Autodesk Inventor part; units mm, degrees
ref_plane "Work Plane1" through (23, 0, 25.5) normal (1, 0, 0) x (0, 0, -1)
ref_plane "YZ Plane" through (0, 0, 0) normal (1, 0, 0) x (0, 1, 0)
ref_plane "XZ Plane" through (0, 0, 0) normal (0, 1, 0) x (-1, 0, 0)
sketch "Sketch1" plane through (0, 0, 0) normal (0, 1, 0) x (-1, 0, 0)
  line L0 (23, 25.5) -> (-23, 25.5)
  line L1 (-23, 25.5) -> (-23, -25.5)
  line L2 (-23, -25.5) -> (23, -25.5)
  line L3 (23, -25.5) -> (23, 25.5)
  point P0 (0, 0)
  point P1 (-23, 0)
  point P2 (23, 0)
  point P3 (0, 25.5)
  point P4 (0, -25.5)
  dimension "d0" = 46
  dimension "d1" = 51
extrude "Extrusion1" add sketch "Sketch1" along normal blind 3
sketch "Sketch2" plane through (0, 3, 0) normal (0, 1, 0) x (1, 0, 0)
  line L0 (-23, -25.5) -> (23, -25.5)
  line L1 (23, 25.5) -> (-23, 25.5)
  line L2 (-23, 25.5) -> (-23, -25.5)
  line L3 (23, -25.5) -> (23, 25.5)
  point P0 (0, 0)
  point P1 (-15, -17.5)
  point P2 (-15, 17.5)
  point P3 (15, -17.5)
  point P4 (15, 17.5)
  dimension "d4" = 8
  dimension "d5" = 8
  dimension "d6" = 8
  dimension "d7" = 8
  dimension "d8" = 8
  dimension "d9" = 8
  dimension "d10" = 8
  dimension "d11" = 8
hole "Hole1" at (-15, 3, 17.5) at (-15, 3, -17.5) at (15, 3, 17.5) at (15, 3, -17.5) direction (0, -1, 0) diameter 2 end through all
ref_plane "Work Plane1" through (23, 0, 25.5) normal (1, 0, 0) x (0, 0, -1)
sketch "Sketch3" plane through (23, 0, 25.5) normal (1, 0, 0) x (0, 0, -1)
  line L0 (25.5, 0) -> (25.5, 200)
  line L1 (60.5, 78.2142) -> (-9.5, 78.2142)
  line L2 (51, 3) -> (0, 3)
  line L3 (0, 3) -> (51, 3)
  line L4 (60.5, 78.2142) -> (60.5, 38.2142)
  line L5 (-9.5, 78.2142) -> (-9.5, 38.2142)
  line L6 (-9.5, 38.2142) -> (0, 3)
  line L7 (60.5, 38.2142) -> (51, 3)
  point P0 (25.5, 78.2142)
  point P1 (25.5, 3)
  point P2 (25.5, 3)
  dimension "d19" = 200
  dimension "d20" = 70
  dimension "d23" = 40
  dimension "d24" = 40
extrude "Extrusion3" add sketch "Sketch3" against normal blind 3
sketch "Sketch4" plane through (20, 0, 25.5) normal (-1, 0, 0) x (0, 0, 1)
  line L0 (-51, 3) -> (0, 3)
  line L1 (-60.5, 78.2142) -> (-60.5, 38.2142)
  line L2 (-51, 3) -> (-60.5, 38.2142)
  line L3 (9.5, 78.2142) -> (-60.5, 78.2142)
  line L4 (-60.5, 38.2142) -> (-60.5, 78.2142)
  line L5 (9.5, 38.2142) -> (9.5, 78.2142)
  line L6 (-60.5, 78.2142) -> (9.5, 78.2142)
  line L7 (0, 3) -> (9.5, 38.2142)
  line L8 (9.5, 78.2142) -> (9.5, 38.2142)
  line L9 (9.5, 38.2142) -> (0, 3)
  line L10 (-47.8927, 3) -> (-57.5, 38.6118)
  line L11 (-57.5, 38.6118) -> (-57.5, 75.2142)
  line L12 (-57.5, 75.2142) -> (6.5, 75.2142)
  line L13 (6.5, 75.2142) -> (6.5, 38.6118)
  line L14 (6.5, 38.6118) -> (-3.1073, 3)
  point P0 (-25.5, 0)
  dimension "d27" = 3
  dimension "d28" = 3
  dimension "d29" = 3
  dimension "d30" = 3
  dimension "d31" = 3
extrude "Extrusion4" add sketch "Sketch4" along normal blind 43 contours L2 L1 L3 L5 L7 L0 L14 L13 L12 L11 L10
equation "\"d27\" = d28"
equation "\"d28\" = d29"
equation "\"d29\" = d30"
equation "\"d30\" = d31"
properties part number "Upper_body_v2"
Build history of the part. All positions in model axes, mm. A direction names the side the tool comes from. Round coordinates to 2 decimals unless told otherwise and drop trailing zeros. Write each loop counter-clockwise with the first axis right and the second up, starting at its lowest first coordinate (ties: lowest second). Pieces come first, ordered by that corner, then holes. Notation, with made-up numbers: (-33.5, -1) -> (19.5, -1) arc R15 cw to (19.5, 18) -> close; hole circle Ø8 at (-24, 78.25). An arc over 180 degrees is marked (long way). Write item = value, one per line.
(1) Band-saw the part on C-C (z = -13). Give the cut face in (x, y), then the cut area to 3 significant figures.
Answer:
outline = (-23, 0) -> (23, 0) -> (23, 78.21) -> (-23, 78.21) -> (-23, 75.21) -> (20, 75.21) -> (20, 3) -> (-23, 3) -> close
area = 493 mm2
(2) Flat gauge pins, fed straight in: pin 1 (1.5 mm diameter, centred on x = 10, z = -10, fed in from -Y); pin 2 (0.9 mm diameter, centred on x = 6.5, y = 1, fed in from +Z); pin 3 (6 mm diameter, centred on y = 55, z = -11, fed in from -X); pin 4 (1.6 mm diameter, centred on x = -15, z = -17.5, fed in from -Y). Where does each tip first touch, or does it go through?
Answer:
pin_1 = 0
pin_2 = 25.5
pin_3 = 20
pin_4 = 75.21
(3) Band-saw the part on A-A (z = 17.5). Give the cut face in (x, y), then the cut area to 3 significant figures.
Answer:
outline = (-23, 0) -> (-16, 0) -> (-16, 3) -> (-23, 3) -> close; (-23, 75.21) -> (20, 75.21) -> (20, 3) -> (16, 3) -> (16, 0) -> (23, 0) -> (23, 78.21) -> (-23, 78.21) -> close; (-14, 0) -> (14, 0) -> (14, 3) -> (-14, 3) -> close
area = 481 mm2
(4) Band-saw the part on B-B (x = 7). Give the cut face in (y, z).
Answer:
outline = (0, -25.5) -> (3, -25.5) -> (38.21, -35) -> (78.21, -35) -> (78.21, 35) -> (38.21, 35) -> (3, 25.5) -> (0, 25.5) -> close; hole (3, -22.39) -> (38.61, -32) -> (75.21, -32) -> (75.21, 32) -> (38.61, 32) -> (3, 22.39) -> close
(5) Band-saw the part on D-D (x = -15). Give the cut face in (y, z).
Answer:
outline = (0, -25.5) -> (3, -25.5) -> (38.21, -35) -> (78.21, -35) -> (78.21, 35) -> (38.21, 35) -> (3, 25.5) -> (0, 25.5) -> (0, 18.5) -> (3, 18.5) -> (3, 22.39) -> (38.61, 32) -> (75.21, 32) -> (75.21, -32) -> (38.61, -32) -> (3, -22.39) -> (3, -18.5) -> (0, -18.5) -> close; (0, -16.5) -> (3, -16.5) -> (3, 16.5) -> (0, 16.5) -> close
(6) Tool access for faces 1 (the face through (-1, 57, 32)), 2 (the face through (0, 1, -25.5)), 3 (the face through (15.89, 1.48, 17.96)): list every direction of +Z, -Z, +X, -X, +Y, -Y with a clear straight run to the whole face (end or side of a thin tool).
Answer:
face_1 = -X
face_2 = -Z, +X, -X, -Y
face_3 = -Y
(7) Probe L1, parallel to X at y = 1.35, z = -17.5; L2, parallel to Z at x = 15, y = 1; L3, parallel to Y at x = -11, z = -18. List the from-to ranges inside material, lowest first.
Answer:
L1 = -23 to -16, -14 to 14, 16 to 23
L2 = -25.5 to -18.5, -16.5 to 16.5, 18.5 to 25.5
L3 = 0 to 3, 75.21 to 78.21
(8) Two-plate mould, pull along Z, no slides. Class faces 4 (the face through (0, 0, 0)), 5 (the face through (0, 58, -35)), 6 (the face through (-1, 57, -32)): pulls with the +Z half, pulls with the -Z half, needs draft (parallel to the pull), parting line crosses it, or undercut.
Answer:
face_4 = needs draft
face_5 = pulls with the -Z half
face_6 = undercut
